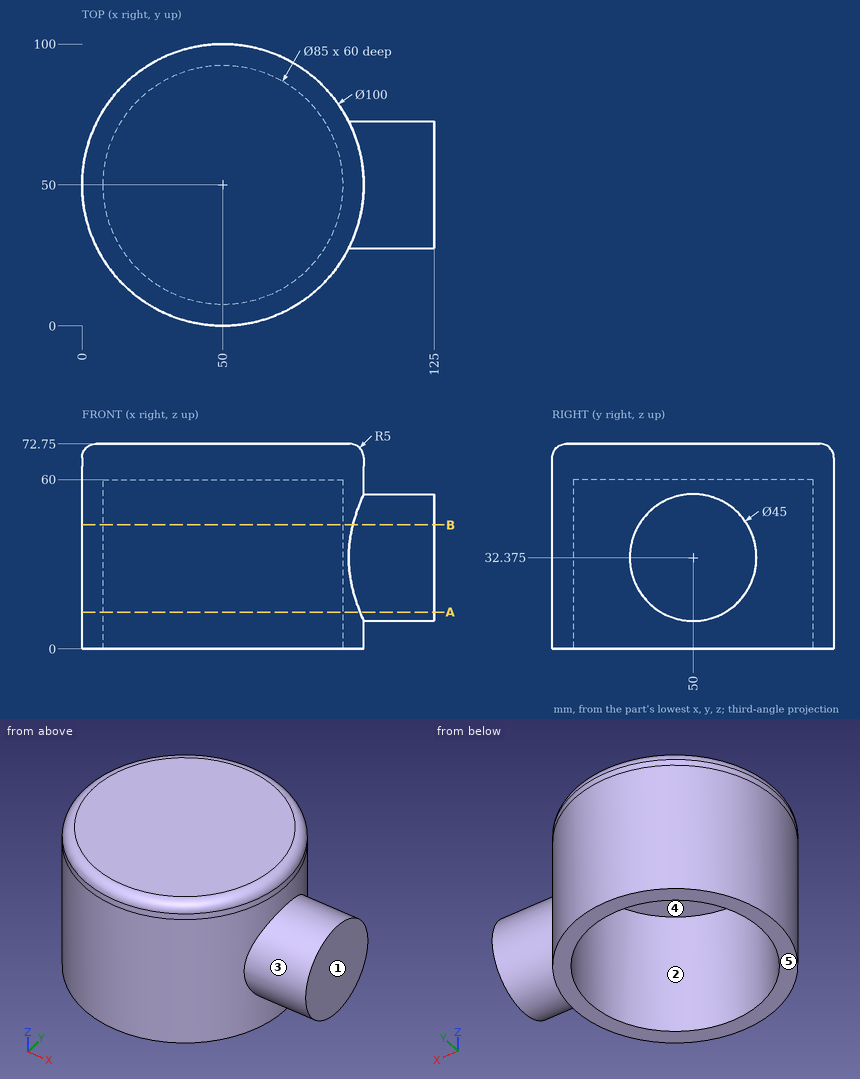
Job drawing, mm, ordinate dimensions from the low corner. One solid piece. A direction names the side the tool comes from. Give positions to 0.01 mm unless a question says otherwise; leave off trailing zeros. Order: outer loops, then holes, each group sorted by start corner. A loop starts at its lowest first (then second) coordinate and runs counter-clockwise, first axis right, second up. Notation, with made-up numbers: (-6.75, -13) -> (26.25, -13) arc R24 ccw to (26.25, 3) -> close; hole circle Ø1 at (86.5, 37). An arc over 180 degrees is marked (long way). Return JSON: item names as keys, results as strings.
Q1. Flat gauge pins, fed straight in: pin 1 (12 mm diameter, centred on x = 68, y = 71.5, fed in from -Z); pin 2 (4 mm diameter, centred on x = 101, z = 29, fed in from -Y); pin 3 (8 mm diameter, centred on x = 95, y = 37, fed in from +Z); pin 4 (4 mm diameter, centred on x = 14, z = 44, fed in from +Y). Where does each tip first touch, or does it go through?
Working result:
{"pin 1": "z = 60", "pin 2": "y = 27.54", "pin 3": "z = 72.75", "pin 4": "y = 86.66"}
Q2. Mould opens along Y. For the marked faces 3, 4 and 5 say: pulls with the +Y half, pulls with the -Y half, needs draft (parallel to the pull), parting line crosses it, or undercut.
Working result:
{"face 3": "parting line crosses it", "face 4": "undercut", "face 5": "needs draft"}
Q3. Drill centre lines: line 1 (Z direction, x = 95, y = 54); line 2 (Y direction, x = 60, z = 27.5); line 3 (X direction, y = 28, z = 11). Where is each one in solid material? Low to high.
Working result:
{"line 1": "0 to 72.75", "line 2": "1.01 to 8.69, 91.31 to 98.99", "line 3": "5.1 to 13.64, 86.36 to 94.9"}
Q4. Saw through at A-A (z = 13). Write the cut outline in (x, y), then the cut area to 3 significant figures.
Working result:
{"outline": "(98.67, 38.56) -> (125, 38.56) -> (125, 61.44) -> (98.67, 61.44) arc R50 ccw (long way) to start; hole circle Ø85 at (50, 50)", "area": "2,760 mm²"}
Q5. Saw through at B-B (z = 44). Write the cut outline in (x, y).
Working result:
{"outline": "(96.14, 30.74) -> (125, 30.74) -> (125, 69.26) -> (96.14, 69.26) arc R50 ccw (long way) to start; hole circle Ø85 at (50, 50)"}
Q6. Which spindle directions (+Z, -Z, +X, -X, +Y, -Y) get a long thin tool onto all of the face, cutting with end or side? Do the marked faces 1 and 2. Say none if no direction does.
Working result:
{"face 1": "+Z, -Z, +X, +Y, -Y", "face 2": "-Z"}
